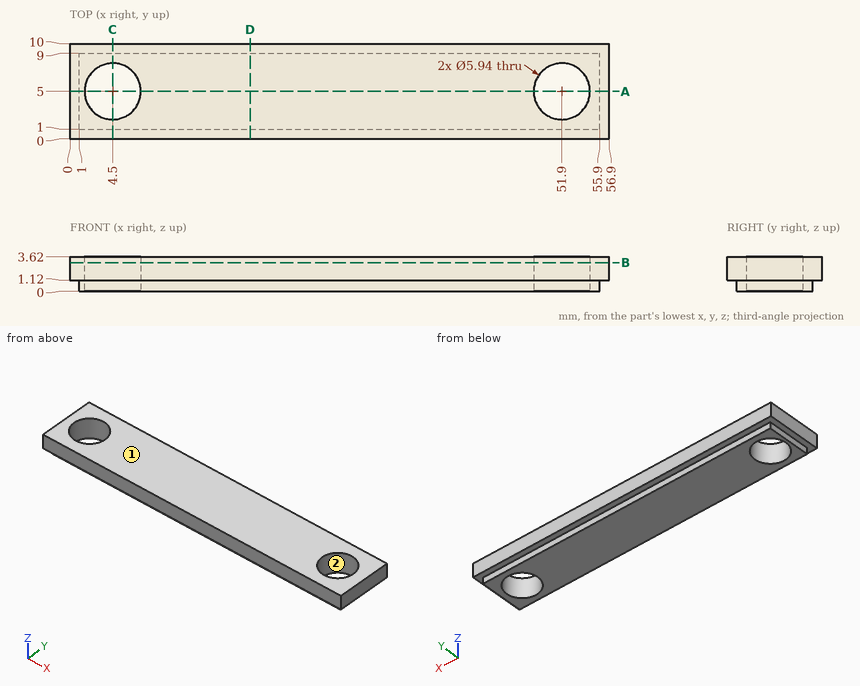
The drawing under review shows one solid part. Ordinate dimensions are in mm from its lowest x, y, z. Give positions to 0.01 mm unless a question says otherwise; leave off trailing zeros. Write each loop counter-clockwise with the first axis right and the second up, starting at its lowest first coordinate (ties: lowest second). Pieces come first, ordered by that corner, then holes. Notation, with made-up numbers: (-27, 20.25) -> (4, 20.25) arc R33 cw to (4, 50.25) -> close; hole circle Ø8 at (-37, -26). An arc over 180 degrees is marked (long way). Put each result on its own line as item: value.
(1) For pin 1 Ø5 at (x, y) = (51.9, 5) entering from -Z; pin 2 Ø0.6 at (y, z) = (6, 0.5) entering from +X; pin 3 Ø0.9 at (x, z) = (41, 0.5) entering from -Y, all flat-tipped, find the tip position at first contact; note any pin that passes through.
Results are:
pin 1: through
pin 2: x = 55.9
pin 3: y = 1
(2) We need section C-C, the plane x = 4.5. Give the boundary of the cut face in (y, z).
Results are:
outline: (0, 1.12) -> (1, 1.12) -> (1, 0) -> (2.03, 0) -> (2.03, 3.62) -> (0, 3.62) -> close; (7.97, 0) -> (9, 0) -> (9, 1.12) -> (10, 1.12) -> (10, 3.62) -> (7.97, 3.62) -> close
(3) To check wall thickness, follow probe 1 along Y at (x, z) = (51.9, 1); probe 2 along X at (y, z) = (6.5, 2.35); probe 3 along X at (y, z) = (6.25, 2.9). State the ranges of each line that lie inside material, in increasing order. Write a range as from..to.
Results are:
probe 1: 1..2.03, 7.97..9
probe 2: 0..1.94, 7.06..49.34, 54.46..56.9
probe 3: 0..1.81, 7.19..49.21, 54.59..56.9
(4) We need section D-D, the plane x = 19. Give the boundary of the cut face in (y, z), and give its area (3 significant figures).
Results are:
outline: (0, 1.12) -> (1, 1.12) -> (1, 0) -> (9, 0) -> (9, 1.12) -> (10, 1.12) -> (10, 3.62) -> (0, 3.62) -> close
area: 34.0 mm²
(5) We need section A-A, the plane y = 5. Give the boundary of the cut face in (x, z).
Results are:
outline: (0, 1.12) -> (1, 1.12) -> (1, 0) -> (1.53, 0) -> (1.53, 3.62) -> (0, 3.62) -> close; (7.47, 0) -> (48.93, 0) -> (48.93, 3.62) -> (7.47, 3.62) -> close; (54.87, 0) -> (55.9, 0) -> (55.9, 1.12) -> (56.9, 1.12) -> (56.9, 3.62) -> (54.87, 3.62) -> close
(6) We need section B-B, the plane z = 3. Give the boundary of the cut face in (x, y), and give its area (3 significant figures).
Results are:
outline: (0, 0) -> (56.9, 0) -> (56.9, 10) -> (0, 10) -> close; hole circle Ø5.94 at (4.5, 5); hole circle Ø5.94 at (51.9, 5)
area: 514 mm²
(7) The part is to be moulded in two halves that separate along Y. For the marked faces 1 and 2, say which applies: pulls with the +Y half, pulls with the -Y half, needs draft (parallel to the pull), parting line crosses it, or undercut.
Results are:
face 1: needs draft
face 2: undercut
